Autodesk Inventor part; units mm, degrees
ref_plane "YZ Plane" through (0, 0, 0) normal (1, 0, 0) x (0, 1, 0)
ref_plane "XZ Plane" through (0, 0, 0) normal (0, 1, 0) x (-1, 0, 0)
sketch "Sketch1" plane through (0, 0, 0) normal (0, 1, 0) x (-1, 0, 0)
  circle A0 centre (0, 0) radius 9.5
  dimension "d0" = 19
extrude "Extrusion1" add sketch "Sketch1" along normal blind 100
ref_plane "Work Plane1" through (0, 0, -9.5) normal (0, 0, 1) x (1, 0, 0)
sketch "Sketch2" plane through (0, 0, -9.5) normal (0, 0, 1) x (1, 0, 0)
  line L0 (0, 0) -> (0, 100)
  line L1 (9.5, 100) -> (-9.5, 100)
  line L2 (0, 50) -> (0, 15)
  line L3 (0, 50) -> (0, 85)
  circle A0 centre (0, 15) radius 5
  circle A1 centre (0, 85) radius 5
  dimension "d4" = 35
  dimension "d5" = 35
  dimension "d6" = 10
  dimension "d7" = 10
extrude "Extrusion2" cut sketch "Sketch2" along normal blind 20
fillet "Fillet1" radius 5 2 edges at (9.5, 100, 0) (9.5, 0, 0)
equation "\"BendRadius\" = Thickness"
equation "\"BendReliefWidth\" = Thickness"
equation "\"BendReliefDepth\" = 0.5 * Thickness"
equation "\"CornerReliefSize\" = 4 * Thickness"
equation "\"MinimumRemnant\" = 2 * Thickness"
equation "\"TransitionRadius\" = BendRadius"
equation "\"JacobiRadiusSize\" = BendRadius"
equation "\"GapSize\" = Thickness"
Can you work these out from the model? Positions are in its coordinate system, mm. Coordinates: 2 decimals unless noted, no trailing zeros. Loops run counter-clockwise (first coordinate to the right, second up) from the corner with the lowest first, then second, coordinate; pieces in that order, holes last. Notation, with made-up numbers: M 77,30.25 L 117,30.25 A23 ccw 117,65.25 Z; hole C 27,82.25 d5. An arc over 180 degrees is marked long. Return JSON: item names as keys, results as strings. Group by question number.
Item 1: Imagine slicing it at D-D (y = 41). Please give me the cut outline in (x, z), and give its area (3 significant figures).
Item 2: Imagine slicing it at A-A (x = 0). Give the number of separate pieces and of enclosed holes in the cut face, and give its area (3 significant figures).
Item 3: Thinking about a two-plate mould opening in Y: for faces 1 (the flat face through (0, 0, 0)), 2 (the flat face through (0, 100, 0)), 3 (the cylindrical face through (-5, 85, 0)), which applies, released by +Y, released by -Y, zero draft, split by the parting line, or undercut?
Item 4: I'm going to push flat-ended pins straight in: pin 1 Ø6 at (y, z) = (54, -6) entering from -X; pin 2 Ø3 at (y, z) = (64, -6.5) entering from +X; pin 3 Ø1.5 at (x, y) = (2.5, 68) entering from -Z. Where does each tip first touch, or does it pass through?
Item 5: If I drill on L1, parallel to Y at x = -3.25, z = -8.5; L2, parallel to Y at x = -3, z = -4.5; L3, parallel to X at y = 15, z = 3.5, over which ranges is the centre line in solid material (lowest first)? Write a range as from..to.
Item 6: Imagine slicing it at C-C (y = 18). Please give me the cut outline in (x, z), and give its area (3 significant figures).
Verdict:
{
 "1": {"outline": "C 0,0 d19", "area": "284 mm^2"},
 "2": {"separate pieces": "3", "enclosed holes": "0", "area": "1,500 mm^2"},
 "3": {"face 1": "released by -Y", "face 2": "released by +Y", "face 3": "undercut"},
 "4": {"pin 1": "stops at x = -9.01", "pin 2": "stops at x = 8.08", "pin 3": "stops at z = -9.34"},
 "5": {"L1": "y = 3.04..11.2, 18.8..81.2, 88.8..96.96", "L2": "y = 0.08..11, 19..81, 89..99.92", "L3": "x = -8.83..-5, 5..8.83"},
 "6": {"outline": "M -4,-8.62 L -4,8.62 A9.5 ccw Z; M 4,-8.62 A9.5 ccw 4,8.62 Z", "area": "136 mm^2"}
}
